Study the drawing (mm; zero at the part's minimum x, y, z) and answer. Round coordinates to 2 decimals unless told otherwise and drop trailing zeros. Write each loop counter-clockwise with the first axis right and the second up, starting at its lowest first coordinate (ties: lowest second). Pieces come first, ordered by that corner, then holes. Notation, with made-up numbers: (-1, -25.5) -> (51, -25.5) arc R18 ccw to (51, 6.5) -> close; hole circle Ø8 at (77.5, 11). An arc over 180 degrees is marked (long way). Return JSON: item names as keys, results as strings.
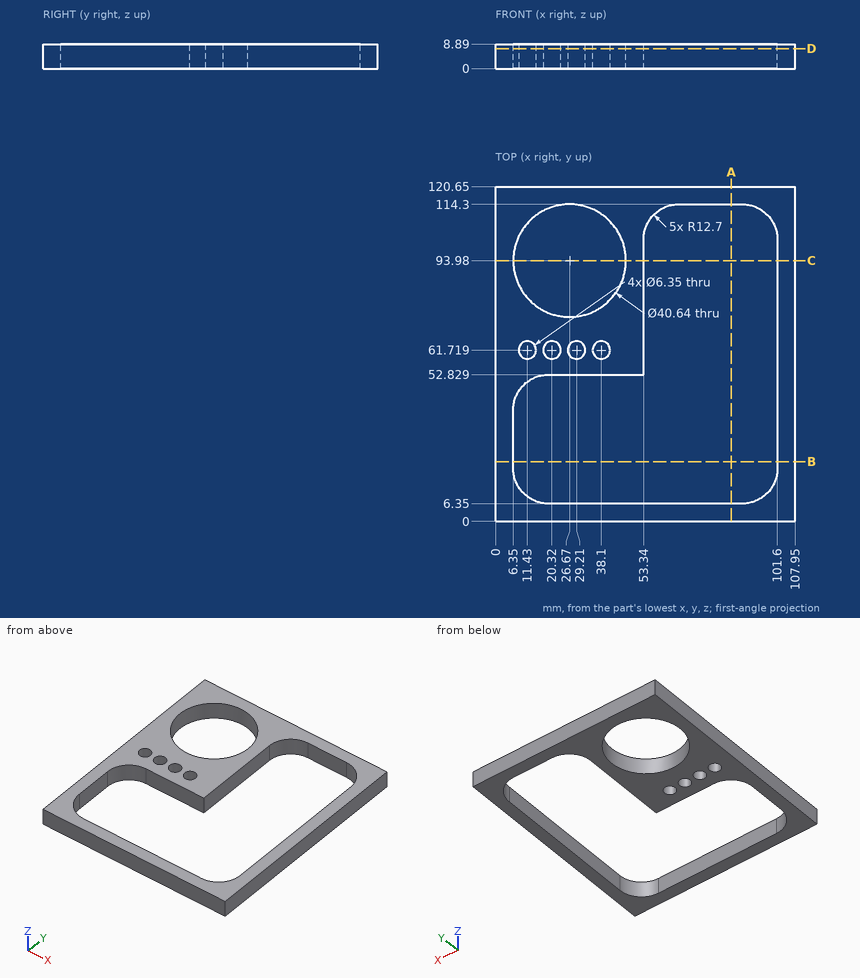
Item 1: Section A-A (x = 85) is taken. Give the vertices of the cut face in (y, z), then the cut area to 3 significant figures.
Worked answers:
{"outline": "(0, 0) -> (6.35, 0) -> (6.35, 8.89) -> (0, 8.89) -> close; (114.3, 0) -> (120.65, 0) -> (120.65, 8.89) -> (114.3, 8.89) -> close", "area": "113 mm2"}
Item 2: Section B-B (y = 21.5) is taken. Give the vertices of the cut face in (x, z), then the cut area to 3 significant figures.
Worked answers:
{"outline": "(0, 0) -> (6.35, 0) -> (6.35, 8.89) -> (0, 8.89) -> close; (101.6, 0) -> (107.95, 0) -> (107.95, 8.89) -> (101.6, 8.89) -> close", "area": "113 mm2"}
Item 3: Section D-D (z = 7.25) is taken. State how many separate pieces and enclosed holes the cut face has, then the cut area to 3 significant figures.
Worked answers:
{"separate pieces": "1", "enclosed holes": "6", "area": "4,380 mm2"}
Item 4: Section C-C (y = 93.98) is taken. Give the vertices of the cut face in (x, z), then the cut area to 3 significant figures.
Worked answers:
{"outline": "(0, 0) -> (6.35, 0) -> (6.35, 8.89) -> (0, 8.89) -> close; (46.99, 0) -> (53.34, 0) -> (53.34, 8.89) -> (46.99, 8.89) -> close; (101.6, 0) -> (107.95, 0) -> (107.95, 8.89) -> (101.6, 8.89) -> close", "area": "169 mm2"}
Item 5: Straight lines are drawn through the part: L1, parallel to X at y = 56, z = 7; L2, parallel to Y at x = 80.5, z = 2; L3, parallel to Y at x = 20.32, z = 6. For each, find the intervals that lie inside material, in ascending order. Write a range as [from, to].
Worked answers:
{"L1": "x = [0, 53.34], [101.6, 107.95]", "L2": "y = [0, 6.35], [114.3, 120.65]", "L3": "y = [0, 6.35], [52.83, 58.54], [64.89, 74.68], [113.28, 120.65]"}
Item 6: A flat-ended cylindrical pin translates along its axis: pin 1 (4.5 mm diameter, centred on y = 59, z = 2.5, fed in from -X). Find the tip coordinate at first contact, or state that the pin passes through.
Worked answers:
{"pin 1": "stops at x = 0"}
